```python
from build123d import *

# Parameters (mm, degrees)
BOSS_EXTRUDE1_DEPTH = 20
BOSS_EXTRUDE1_DRAFT = -0.5
FILLET1_R           = 1
FILLET2_R           = 2


with BuildPart() as part:
    # Sketch1 → Boss-Extrude1 (with draft: the straight prism first)
    with BuildSketch(Plane.XY):
        Polygon((-4, 12.190598923), (-4, -12.190598923), (0, -14.5), (0, 14.5), align=None)
    extrude(amount=-BOSS_EXTRUDE1_DEPTH)
    # Boss-Extrude1: the draft: its side faces are tilted about the plane it starts from
    boss_extrude1_sides = [part.faces().sort_by_distance(p)[0] for p in [
        (-4, 0, -10),
        (-2, -13.345299462, -10),
        (0, 0, -10),
        (-2, 13.345299462, -10),
    ]]
    draft(boss_extrude1_sides, Plane.XY, BOSS_EXTRUDE1_DRAFT)

    # Fillet1
    fillet1_edges = [part.edges().sort_by_distance(p)[0] for p in [
        (-2, 13.143761083, -20),
        (-3.825462644, 0, -20),
        (-2, -13.143761083, -20),
        (-4, 0, 0),
        (-2, 13.345299462, 0),
        (0, 0, 0),
        (-2, -13.345299462, 0),
        (-3.912731322, -12.140214329, -10),
        (-3.912731322, 12.140214329, -10),
        (-0.087268678, 14.348846216, -10),
        (-0.087268678, -14.348846216, -10),
        (-0.174537356, 0, -20),
    ]]
    fillet(fillet1_edges, radius=FILLET1_R)

    # Sketch2 → Cut-Revolve1 (revolve, cut)
    with BuildSketch(Plane(origin=(0, 0, 0), x_dir=(1, 0, 0), z_dir=(0, 1, 0))):
        with BuildLine():
            Line((8.726833455, 10.000724303), (8.726833455, -0.726109151))
            ThreePointArc((8.726833455, -0.726109151), (16.311850131, 2.415707627), (19.453666909, 10.000724303))
            ThreePointArc((19.453666909, 10.000724303), (16.311850131, 17.58574098), (8.726833455, 20.727557758))
            Line((8.726833455, 20.727557758), (8.726833455, 10.000724303))
        make_face()
    revolve(axis=Axis((8.726833455, 0, -20.727557758), (0, 0, 1)), mode=Mode.SUBTRACT)

    # Fillet2
    fillet2_edges = [part.edges().sort_by_distance(p)[0] for p in [
        (-0.139958798, 0, -16.037689693),
    ]]
    fillet(fillet2_edges, radius=FILLET2_R)


solid = part.part
```
Part model, mm, in its own coordinate system. A direction names the side the tool comes from. Round coordinates to 2 decimals unless told otherwise and drop trailing zeros. Order: outer loops, then holes, each group sorted by start corner. A loop starts at its lowest first (then second) coordinate and runs counter-clockwise, first axis right, second up. Notation, with made-up numbers: M 31,-10.5 L 81,-10.5 A20 cw 81,28.5 Z; hole C 87,20.5 d5. An arc over 180 degrees is marked long. Answer in a Markdown table with one row per item. Add a question column.
Q1. Cut at A-A on y = -8.25. Give the cut face in (x, z).
Q2. Wall check: L1, parallel to Z at x = -2.9, y = -2.5; L2, parallel to Z at x = -1.15, y = 0.75; L3, parallel to X at y = 12.25, z = -5.25. Give the ranges that are in metal, low to high. Write a range as from..to.
Q3. 3-axis set-ups, long thin cutter, end or side, ignore diameter. For faces 1 (the face through (-3.78, 12.06, -10.14)), 2 (the face through (-0.576, 13.473, -10.143)), 3 (the face through (-0.601, -13.488, -10.143)), 4 (the face through (-3.78, -12.06, -10.14)): which of +Z, -Z, +X, -X, +Y, -Y reach the whole face in a straight line?
Q4. Pin check, flat tips, straight feed: pin 1 (2 mm diameter, centred on x = -3, y = 2, fed in from +Z); pin 2 (4 mm diameter, centred on y = -11, z = -4, fed in from -X); pin 3 (5 mm diameter, centred on y = 8, z = -15.5, fed in from +X); pin 4 (6 mm diameter, centred on y = -2, z = -16.5, fed in from -X). Stop position of each tip, or through.
Established:
| question | item | result |
|---|---|---|
| 1 | outline | M -3.99,-1.01 L -3.83,-19.01 A1 ccw -2.83,-20 L -1.17,-20 A1 ccw -0.17,-19.01 L -0.01,-1.01 A1 ccw -1.01,0 L -2.99,0 A1 ccw Z |
| 2 | L1 | z = -20..0 |
| 2 | L2 | z = -20..-14.12, -5.88..0 |
| 2 | L3 | x = -3.7..-0.05 |
| 3 | face 1 | -Z, -X, +Y |
| 3 | face 2 | -Z, +Y |
| 3 | face 3 | -Z, -Y |
| 3 | face 4 | -Z, -X, -Y |
| 4 | pin 1 | stops at z = 0 |
| 4 | pin 2 | stops at x = -3.98 |
| 4 | pin 3 | stops at x = -0.11 |
| 4 | pin 4 | stops at x = -3.88 |
